from build123d import *

# Parameters (mm, degrees)
EXTRUDE_1_DEPTH     = 4
CUT_EXTRUDE_1_REACH = 18.86
SKETCH_2_R          = 2.5


with BuildPart() as part:
    # 草图1 → 凸台-拉伸1 (new body)
    with BuildSketch(Plane(origin=(0, 0, 0), x_dir=(1, 0, 0), z_dir=(0, 1, 0))):
        with BuildLine():
            Line((3.479852727, 0.375), (1.988487272, 14.214285714))
            ThreePointArc((1.988487272, 14.214285714), (0, 16), (-1.988487272, 14.214285714))
            Line((-1.988487272, 14.214285714), (-3.479852727, 0.375))
            ThreePointArc((-3.479852727, 0.375), (0, -3.5), (3.479852727, 0.375))
        make_face()
    extrude(amount=EXTRUDE_1_DEPTH)

    # 草图2 → 切除-拉伸1 (cut, up to next)
    with BuildSketch(Plane(origin=(0, 4, 0), x_dir=(1, 0, 0), z_dir=(0, 1, 0)), mode=Mode.PRIVATE) as cut_extrude_1_sk1:
        with Locations(Location((0, 0, 0), (0, 0, 270))):
            Circle(SKETCH_2_R)
    cut_extrude_1_tool1 = extrude(cut_extrude_1_sk1.sketch, amount=-CUT_EXTRUDE_1_REACH, mode=Mode.PRIVATE) & part.part
    add(cut_extrude_1_tool1.solids().sort_by_distance((0, 4, 0))[0], mode=Mode.SUBTRACT)


solid = part.part
Source: CAD feature listing. Evaluate the final solid. Frame: model axes, mm. Coordinates: 2 decimals unless noted, no trailing zeros. Loops run counter-clockwise (first coordinate to the right, second up) from the corner with the lowest first, then second, coordinate; pieces in that order, holes last. Notation, with made-up numbers: (34, -37) - (61, -37) arc R8 ccw to (61, -28) - close; hole circle Ø3 at (81, 65.25). An arc over 180 degrees is marked (long way). One line per item, written item: value. Start each with the question number.
1. Section D-D (z = -5.75). Return the cut outline in (x, y), and give its area (3 significant figures).
2. Section A-A (x = 0). Return the cut outline in (y, z), and give its area (3 significant figures).
3. Mould query, pull axis Z, two halves, no side actions, for faces 1 (the flat face through (2.745, 1.972, -7.198)), 2 (the cylindrical face through (-2.44, 2.03, -0.54)), 3 (the flat face through (0, 0, -6)). Classes: pulls with the +Z half, pulls with the -Z half, needs draft (parallel to the pull), parting line crosses it, or undercut.
4. Section B-B (z = 0). Return the cut outline in (x, y), and give its area (3 significant figures).
5. Contact query for a flat-ended pin moving along its axis: P1, Ø1, axis at x = 1.5, y = 0.5, coming from the +Z side. Output: stop coordinate, or through.
6. Section C-C (y = 0.7). Return the cut outline in (x, z) (3 decimals).
7. Ray query, L1, parallel to X at y = 3.2, z = 0; L2, parallel to Z at x = 1.25, y = 1.9; L3, parallel to Z at x = 0.25, y = 0.95. Return the intervals inside material, ascending.
Verdict:
1. outline: (-2.9, 0) - (2.9, 0) - (2.9, 4) - (-2.9, 4) - close
1. area: 23.2 mm2
2. outline: (0, -16) - (4, -16) - (4, -2.5) - (0, -2.5) - close; (0, 2.5) - (4, 2.5) - (4, 3.5) - (0, 3.5) - close
2. area: 58.0 mm2
3. face 1: pulls with the -Z half
3. face 2: undercut
3. face 3: needs draft
4. outline: (-3.5, 0) - (-2.5, 0) - (-2.5, 4) - (-3.5, 4) - close; (2.5, 0) - (3.5, 0) - (3.5, 4) - (2.5, 4) - close
4. area: 8.00 mm2
5. P1: stops at z = 3.35
6. outline: (-3.48, -0.375) - (-1.988, -14.214) arc R2 ccw to (1.988, -14.214) - (3.48, -0.375) arc R3.5 ccw (long way) to start; hole circle Ø5 at (0, 0)
7. L1: x = -3.5 to -2.5, 2.5 to 3.5
7. L2: z = -15.56 to -2.17, 2.17 to 3.27
7. L3: z = -15.98 to -2.49, 2.49 to 3.49
